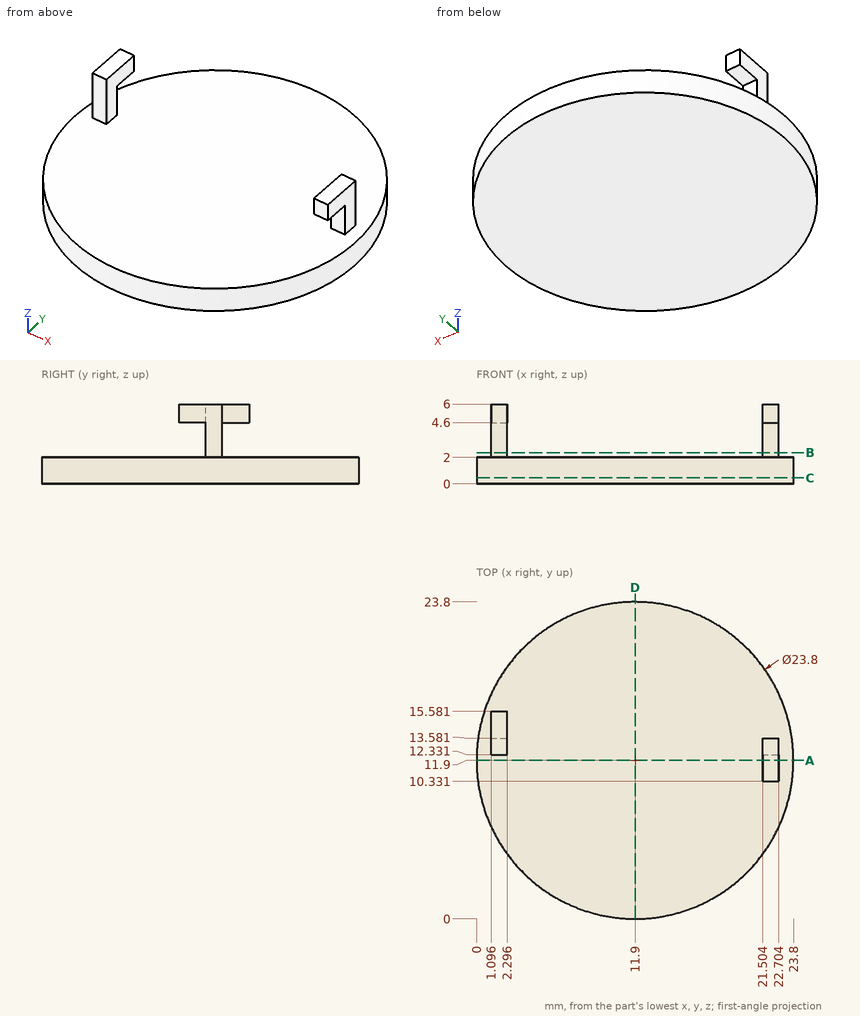
Drawing for the job (mm, zero at the part's lowest x, y, z). Round coordinates to 2 decimals unless told otherwise and drop trailing zeros. Write each loop counter-clockwise with the first axis right and the second up, starting at its lowest first coordinate (ties: lowest second). Pieces come first, ordered by that corner, then holes. Notation, with made-up numbers: M 15,87 L 74,87 A24 ccw 74,111 Z; hole C 71,62 d11. An arc over 180 degrees is marked long. One line per question, with ' | ' between items.
1. Cut at C-C on z = 0.45. Write the cut outline in (x, y), and give its area (3 significant figures).
Working result:
outline: C 11.9,11.9 d23.8 | area: 445 mm2
2. Cut at B-B on z = 2.35. Write the cut outline in (x, y).
Working result:
outline: M 1.1,12.33 L 2.3,12.33 L 2.3,13.58 L 1.1,13.58 Z; M 21.5,12.33 L 22.7,12.33 L 22.7,13.58 L 21.5,13.58 Z
3. Cut at D-D on x = 11.9. Write the cut outline in (y, z).
Working result:
outline: M 0,0 L 23.8,0 L 23.8,2 L 0,2 Z
4. Pin check, flat tips, straight feed: pin 1 Ø3 at (x, y) = (6, 14.5) entering from +Z; pin 2 Ø2.5 at (y, z) = (13.5, 5) entering from +X; pin 3 Ø0.6 at (x, z) = (1.5, 5.5) entering from +Y. Stop position of each tip, or through.
Working result:
pin 1: z = 2 | pin 2: x = 22.7 | pin 3: y = 15.58
5. Cut at A-A on y = 11.9. Write the cut outline in (x, z).
Working result:
outline: M 0,0 L 23.8,0 L 23.8,2 L 0,2 Z; M 21.5,4.6 L 22.7,4.6 L 22.7,6 L 21.5,6 Z
6. Probe L1, parallel to Z at x = 3.75, y = 11.25; L2, parallel to X at y = 1.5, z = 0.7 (1 decimal); L3, parallel to Y at x = 2.25, z = 3.8. List the from-to ranges inside material, lowest first. Write a range as from..to.
Working result:
L1: 0..2 | L2: 6.1..17.7 | L3: 12.33..13.58
